For this review, use the dimensioned drawing (mm, ordinates from the lowest corner) and the shaded views. A direction names the side the tool comes from. Give positions to 0.01 mm unless a question says otherwise; leave off trailing zeros. Write each loop counter-clockwise with the first axis right and the second up, starting at its lowest first coordinate (ties: lowest second). Pieces come first, ordered by that corner, then holes.
1) Draft analysis for pull direction Y (two halves, no side actions). For the marked faces 1, 2, 3 and 4, state which applies: pulls with the +Y half, pulls with the -Y half, needs draft (parallel to the pull), parting line crosses it, or undercut.
2) Machinability: for the marked faces 5 and 6, which of the approach directions +Z, -Z, +X, -X, +Y, -Y give a long, thin tool a straight path to every point of the face, cutting with its end or side? Answer none if there is none.
3) For P1, Ø14, axis at x = 19, y = 14.5, coming from the +Z side; P2, Ø1.5, axis at x = 19.5, y = 22, coming from the +Z side, all flat-tipped, find the tip position at first contact; note any pin that passes through.
4) Wall thickness on line 1 along Y through (x, z) = (25, 0.85); line 2 along X through (y, z) = (41.5, 6): over which ranges is each line inside the solid? List them lowest first.
5) We need section C-C on z = 5.75. Give the boundary of the cut face in (x, y).
6) We need section A-A on y = 25. Give the boundary of the cut face in (x, z).
7) We need section D-D on x = 7. Give the boundary of the cut face in (y, z).
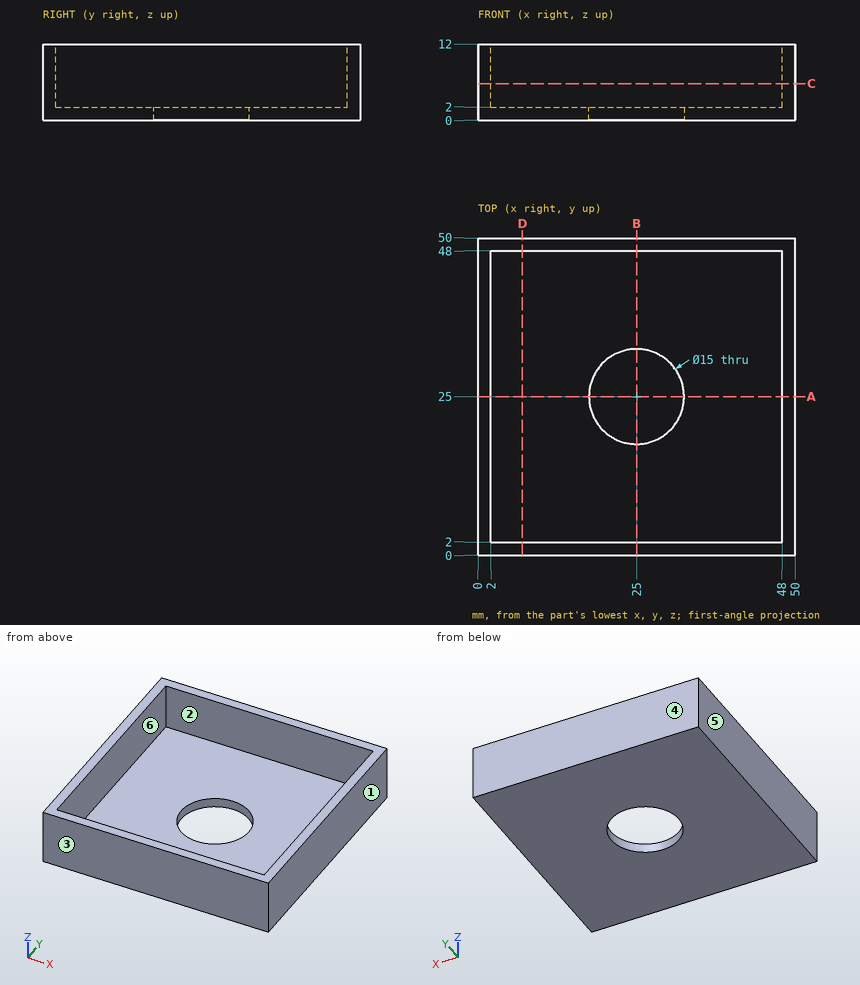
Results list:
1. face 1: needs draft
1. face 2: undercut
1. face 3: pulls with the -Y half
1. face 4: pulls with the +Y half
2. face 5: +Z, -Z, -X, +Y, -Y
2. face 6: +Z
3. P1: stops at z = 2
3. P2: passes through
4. line 1: y = 0 to 17.5, 32.5 to 50
4. line 2: x = 0 to 2, 48 to 50
5. outline: (0, 0) - (50, 0) - (50, 50) - (0, 50) - close; hole (2, 2) - (48, 2) - (48, 48) - (2, 48) - close
6. outline: (0, 0) - (17.5, 0) - (17.5, 2) - (2, 2) - (2, 12) - (0, 12) - close; (32.5, 0) - (50, 0) - (50, 12) - (48, 12) - (48, 2) - (32.5, 2) - close
7. outline: (0, 0) - (50, 0) - (50, 12) - (48, 12) - (48, 2) - (2, 2) - (2, 12) - (0, 12) - close
